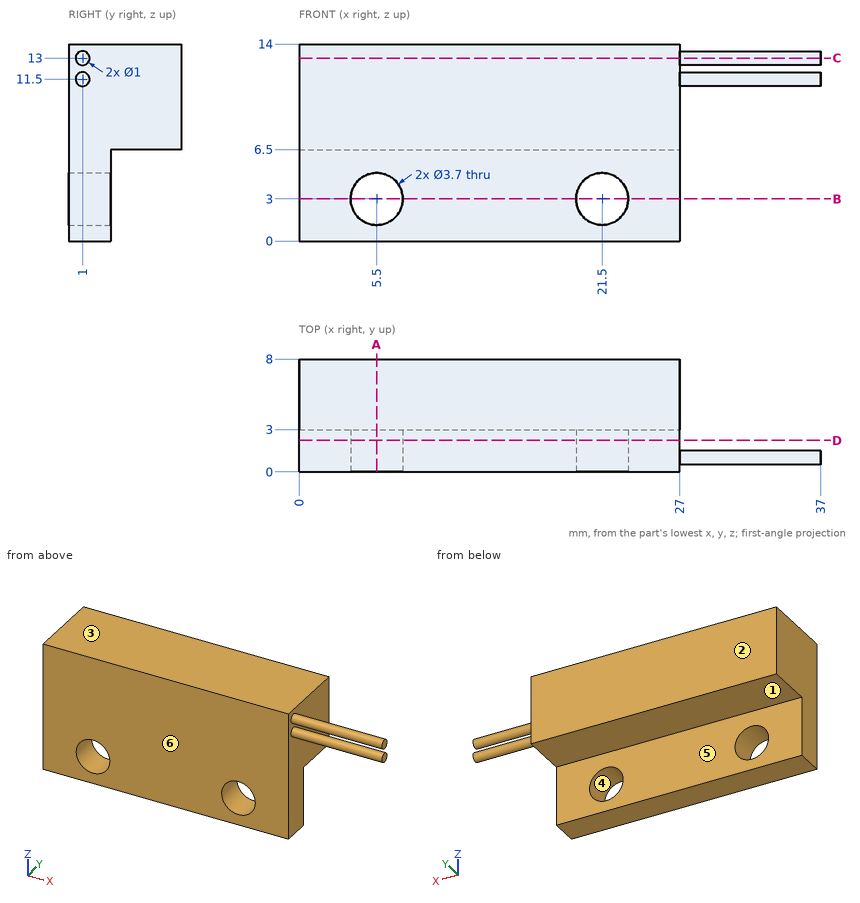
Study the drawing (mm; zero at the part's minimum x, y, z) and answer. A direction names the side the tool comes from. Round coordinates to 2 decimals unless told otherwise and drop trailing zeros. Loops run counter-clockwise (first coordinate to the right, second up) from the corner with the lowest first, then second, coordinate; pieces in that order, holes last. Notation, with made-up numbers: (81, 79.25) - (110, 79.25) arc R16 ccw to (110, 107.25) - close; hole circle Ø7 at (59.25, 1.5). An arc over 180 degrees is marked (long way). Use one line per item in the form item = value. Start each with the question number.
1. A tool of negligible diameter and unlimited length cuts with its end or side. For the marked faces 5 and 6, from which of +Z, -Z, +X, -X, +Y, -Y can it reach the whole face along a straight path? Write none if from no direction.
2. Given pin 1 Ø3 at (x, z) = (21.5, 3) entering from -Y; pin 2 Ø4 at (y, z) = (5, 7.5) entering from +X; pin 3 Ø2.5 at (x, y) = (15.5, 4.5) entering from -Z; pin 4 Ø5 at (x, z) = (18, 3) entering from +Y, each flat-ended and moving along its own axis, determine where each tip first touches the part or whether it passes through.
3. The part is cut by section B-B on z = 3. Determine the outline of the cut face in (x, y), then the cut area to 3 significant figures.
4. Consider line 1 (X direction, y = 1, z = 3); line 2 (Z direction, x = 5.5, y = 2.2); line 3 (Y direction, x = 7.5, z = 3.5). Determine where each line is inside the solid, lowest interval first. Write a range as [from, to].
5. The part is cut by section D-D on y = 2.25. Determine the outline of the cut face in (x, z), then the cut area to 3 significant figures.
6. The part is cut by section A-A on x = 5.5. Determine the outline of the cut face in (y, z), then the cut area to 3 significant figures.
7. The part is cut by section C-C on z = 13. Determine the outline of the cut face in (x, y), then the cut area to 3 significant figures.
8. For a pull along Z with two mould halves and no side action, classify the marked faces 1, 2, 3 and 4 as pulls with the +Z half, pulls with the -Z half, needs draft (parallel to the pull), parting line crosses it, or undercut.
Geometry check:
q1.face_5 = -Z, +X, -X, +Y
q1.face_6 = +Z, -Z, +X, -X, -Y
q2.pin_1 = through
q2.pin_2 = 27
q2.pin_3 = 6.5
q2.pin_4 = 3
q3.outline = (0, 0) - (3.65, 0) - (3.65, 3) - (0, 3) - close; (7.35, 0) - (19.65, 0) - (19.65, 3) - (7.35, 3) - close; (23.35, 0) - (27, 0) - (27, 3) - (23.35, 3) - close
q3.area = 58.8 mm^2
q4.line_1 = [0, 3.65], [7.35, 19.65], [23.35, 27]
q4.line_2 = [0, 1.15], [4.85, 14]
q4.line_3 = [0, 3]
q5.outline = (0, 0) - (27, 0) - (27, 14) - (0, 14) - close; hole circle Ø3.7 at (5.5, 3); hole circle Ø3.7 at (21.5, 3)
q5.area = 356 mm^2
q6.outline = (0, 0) - (3, 0) - (3, 1.15) - (0, 1.15) - close; (0, 4.85) - (3, 4.85) - (3, 6.5) - (8, 6.5) - (8, 14) - (0, 14) - close
q6.area = 68.4 mm^2
q7.outline = (0, 0) - (27, 0) - (27, 0.5) - (37, 0.5) - (37, 1.5) - (27, 1.5) - (27, 8) - (0, 8) - close
q7.area = 226 mm^2
q8.face_1 = pulls with the -Z half
q8.face_2 = needs draft
q8.face_3 = pulls with the +Z half
q8.face_4 = undercut
